from build123d import *

# Parameters (mm, degrees)
SKETCH1_R                = 6.9
SKETCH1_R_2              = 4.9
BOSS_EXTRUDE1_DEPTH      = 38
SKETCH2_R                = 7.5
SKETCH2_R_2              = 6.9
BOSS_EXTRUDE2_DEPTH      = 20.5
BOSS_EXTRUDE3_REACH      = 22.5
BOSS_EXTRUDE3_END_RADIUS = 7.5
BOSS_EXTRUDE3_START      = 13
SKETCH3_W                = 10.5
SKETCH3_H                = 15
CUT_EXTRUDE1_START       = -2.5
CUT_EXTRUDE1_DEPTH       = 2.5
SKETCH5_R                = 1.6
CUT_EXTRUDE2_DEPTH       = 10


with BuildPart() as part:
    # Sketch1 → Boss-Extrude1 (new body)
    with BuildSketch(Plane(origin=(0, 0, 0), x_dir=(1, 0, 0), z_dir=(0, 1, 0))):
        with Locations(Location((0, 0, 0), (0, 0, 270))):  # turned: the seam where the file's is
            Circle(SKETCH1_R)
        with Locations(Location((0, 0, 0), (0, 0, 270))):  # turned: the seam where the file's is
            Circle(SKETCH1_R_2, mode=Mode.SUBTRACT)
    extrude(amount=-BOSS_EXTRUDE1_DEPTH)

    # Sketch2 → Boss-Extrude2 (add, through all)
    with BuildSketch(Plane(origin=(0, -17.5, 0), x_dir=(-1, 0, 0), z_dir=(0, -1, 0))):
        with Locations(Location((0, 0, 0), (0, 0, 90))):  # turned: the seam where the file's is
            Circle(SKETCH2_R)
        with Locations(Location((0, 0, 0), (0, 0, 270))):  # turned: the seam where the file's is
            Circle(SKETCH2_R_2, mode=Mode.SUBTRACT)
    extrude(amount=BOSS_EXTRUDE2_DEPTH)

    # Boss-Extrude3: up to this cylinder (the profile starts outside it)
    boss_extrude3_end = Plane(origin=(0, -30.5, 0), z_dir=(0, 1, 0)) * Cylinder(BOSS_EXTRUDE3_END_RADIUS, 61, mode=Mode.PRIVATE)
    # Sketch3 → Boss-Extrude3 (add, up to the surface)
    with BuildSketch(Plane.XY.offset(BOSS_EXTRUDE3_START), mode=Mode.PRIVATE) as boss_extrude3_sk1:
        with Locations((0, -30.5)):
            Rectangle(SKETCH3_W, SKETCH3_H)
    boss_extrude3_tool1 = extrude(boss_extrude3_sk1.sketch, amount=-BOSS_EXTRUDE3_REACH, mode=Mode.PRIVATE) - boss_extrude3_end
    add(boss_extrude3_tool1.solids().sort_by_distance((0, -30.5, 13))[0])

    # Sketch4 → Cut-Extrude1 (cut)
    with BuildSketch(Plane.XY.offset(13).offset(CUT_EXTRUDE1_START)):
        with BuildLine():
            Line((-3.1, -23), (-3.1, -29.75))
            ThreePointArc((-3.1, -29.75), (0, -32.85), (3.1, -29.75))
            Line((3.1, -29.75), (3.1, -23))
            Line((3.1, -23), (-3.1, -23))
        make_face()
    extrude(amount=-CUT_EXTRUDE1_DEPTH, mode=Mode.SUBTRACT)

    # Sketch5 → Cut-Extrude2 (cut)
    with BuildSketch(Plane.XY.offset(13)):
        with Locations((0, -29.75)):
            Circle(SKETCH5_R)
    extrude(amount=-CUT_EXTRUDE2_DEPTH, mode=Mode.SUBTRACT)


solid = part.part
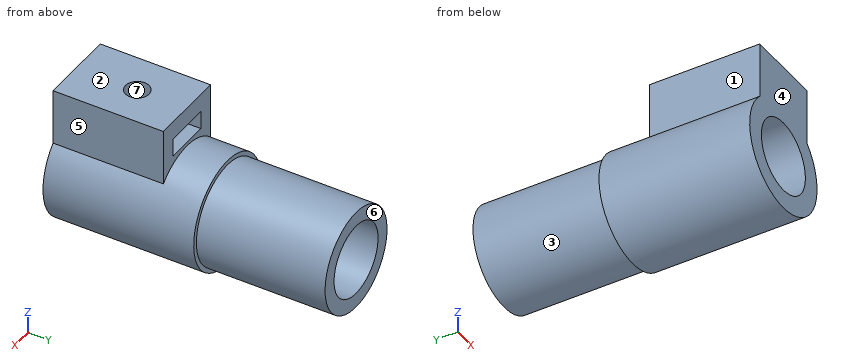
Part model, mm, in its own coordinate system. Face numbers are marked on the shaded views. A direction names the side the tool comes from. Coordinates: 2 decimals unless noted, no trailing zeros. Loops run counter-clockwise (first coordinate to the right, second up) from the corner with the lowest first, then second, coordinate; pieces in that order, holes last. Notation, with made-up numbers: (69.25, 68) -> (87.25, 68) arc R8 ccw to (87.25, 74) -> close; hole circle Ø3 at (17.25, 81.25). An arc over 180 degrees is marked (long way). Use a Markdown table: item, result. Add a question column.
Item 1: Flat gauge pins, fed straight in: P1, Ø5, axis at x = -3, y = -17, coming from the -Z side; P2, Ø6, axis at y = -33.5, z = 11, coming from the -X side; P3, Ø12, axis at y = -12, z = 7.5, coming from the -X side (3 decimals). Where does each tip first touch, or does it go through?
Item 2: Pull direction Y, two halves, no side cores. Call the marked faces 4, 5, 6 and 7: +Y half, -Y half, draft (parallel to the pull), parting line (faces both ways), or undercut.
Item 3: Probe probe 1 along Z at (x, y) = (2.25, -26); probe 2 along Y at (x, z) = (0, 11.8); probe 3 along Z at (x, y) = (-0.5, -27). List the from-to ranges inside material, lowest first.
Item 4: Band-saw the part on B-B on x = 0. Write the cut outline in (y, z), plus the area to 3 significant figures.
Item 5: Band-saw the part on C-C on z = 0. Write the cut outline in (x, y).
Item 6: Band-saw the part on A-A on y = -23.5. Write the cut outline in (x, z).
Item 7: Band-saw the part on D-D on x = -4.25. Write the cut outline in (y, z), plus the area to 3 significant figures.
Item 8: Which spindle directions (+Z, -Z, +X, -X, +Y, -Y) get a long thin tool onto all of the face, cutting with end or side? Do the marked faces 1, 2 and 3. Say none if no direction does.
Geometry says:
| question | item | result |
|---|---|---|
| 1 | P1 | z = -7.48 |
| 1 | P2 | x = -5.25 |
| 1 | P3 | x = -6.735 |
| 2 | face 4 | -Y half |
| 2 | face 5 | draft |
| 2 | face 6 | +Y half |
| 2 | face 7 | undercut |
| 3 | probe 1 | -7.15 to -4.35, 4.35 to 8, 10.5 to 13 |
| 3 | probe 2 | -38 to -31.35, -28.15 to -23 |
| 3 | probe 3 | -7.48 to -4.87, 4.87 to 8, 10.5 to 13 |
| 4 | outline | (-38, -7.5) -> (-17.5, -7.5) -> (-17.5, -6.9) -> (0, -6.9) -> (0, -4.9) -> (-38, -4.9) -> close; (-38, 4.9) -> (-31.35, 4.9) -> (-31.35, 8) -> (-32.85, 8) -> (-32.85, 10.5) -> (-31.35, 10.5) -> (-31.35, 13) -> (-38, 13) -> close; (-28.15, 4.9) -> (0, 4.9) -> (0, 6.9) -> (-17.5, 6.9) -> (-17.5, 7.5) -> (-23, 7.5) -> (-23, 8) -> (-28.15, 8) -> close; (-28.15, 10.5) -> (-23, 10.5) -> (-23, 13) -> (-28.15, 13) -> close |
| 4 | area | 217 mm² |
| 5 | outline | (-7.5, -38) -> (-4.9, -38) -> (-4.9, 0) -> (-6.9, 0) -> (-6.9, -17.5) -> (-7.5, -17.5) -> close; (4.9, -38) -> (7.5, -38) -> (7.5, -17.5) -> (6.9, -17.5) -> (6.9, 0) -> (4.9, 0) -> close |
| 6 | outline | (-5.25, 5.36) arc R7.5 ccw (long way) to (5.25, 5.36) -> (5.25, 13) -> (-5.25, 13) -> close; hole circle Ø9.8 at (0, 0); hole (-3.1, 8) -> (3.1, 8) -> (3.1, 10.5) -> (-3.1, 10.5) -> close |
| 7 | outline | (-38, -6.18) -> (-17.5, -6.18) -> (-17.5, -5.44) -> (0, -5.44) -> (0, -2.44) -> (-38, -2.44) -> close; (-38, 2.44) -> (0, 2.44) -> (0, 5.44) -> (-17.5, 5.44) -> (-17.5, 6.18) -> (-23, 6.18) -> (-23, 13) -> (-38, 13) -> close |
| 7 | area | 361 mm² |
| 8 | face 1 | +Z, -X, +Y, -Y |
| 8 | face 2 | +Z, +X, -X, +Y, -Y |
| 8 | face 3 | +Y |
